The model under review builds one solid part; all positions refer to its coordinate system, in mm. A direction names the side the tool comes from. Coordinates: 2 decimals unless noted, no trailing zeros. Loops run counter-clockwise (first coordinate to the right, second up) from the corner with the lowest first, then second, coordinate; pieces in that order, holes last. Notation, with made-up numbers: M 8.25,80.5 L 58.25,80.5 A22 ccw 58.25,100.5 Z; hole C -18,89.25 d6. An arc over 180 degrees is marked long. Return JSON: item names as keys, results as strings.
```python
from build123d import *

# Parameters (mm, degrees)
SZKIC1_R                    = 7
DODANIE_WYCI_GNI_CIE1_DEPTH = 28
WYTNIJ_WYCI_GNI_CIE1_DEPTH  = 30.69848481


with BuildPart() as part:
    # Szkic1 → Dodanie-wyciągnięcie1 (new body)
    with BuildSketch(Plane.XY):
        Circle(SZKIC1_R)
        Polygon((4.922995461, 0.874137115), (1.704472782, 4.700507689), (-3.218522678, 3.826370574), (-4.922995461, -0.874137115), (-1.704472782, -4.700507689), (3.218522678, -3.826370574), align=None, mode=Mode.SUBTRACT)
    extrude(amount=DODANIE_WYCI_GNI_CIE1_DEPTH)

    # Szkic2 → Wytnij-wyciągnięcie1 (cut, through all)
    with BuildSketch(Plane.XY.offset(28)):
        Polygon((-3.423048557, 4.978226449), (1.499946904, 5.852363564), (1.23770577, 7.329262202), (-3.685289691, 6.455125087), align=None)
    extrude(amount=-WYTNIJ_WYCI_GNI_CIE1_DEPTH, mode=Mode.SUBTRACT)


solid = part.part
```
1. To check wall thickness, follow line 1 (Y direction, x = 0.5, z = 21.5); line 2 (X direction, y = -3.5, z = 13); line 3 (Y direction, x = 2.25, z = 9.5). State the ranges of each line that lie inside material, in increasing order.
Check values:
{"line 1": "-6.98 to -4.31, 4.49 to 5.67", "line 2": "-6.06 to -2.71, 3.34 to 6.06", "line 3": "-6.63 to -4, 4.05 to 6.63"}
2. Add section C-C on y = 1.25. Give the boundary of the cut face in (x, z).
Check values:
{"outline": "M -6.89,0 L -4.15,0 L -4.15,28 L -6.89,28 Z; M 4.61,0 L 6.89,0 L 6.89,28 L 4.61,28 Z"}
3. Add section B-B on x = 0. Give the boundary of the cut face in (y, z), plus the area to 3 significant figures.
Check values:
{"outline": "M -7,0 L -4.4,0 L -4.4,28 L -7,28 Z; M 4.4,0 L 5.59,0 L 5.59,28 L 4.4,28 Z", "area": "106 mm²"}
4. Add section A-A on z = 4. Give the boundary of the cut face in (x, y).
Check values:
{"outline": "M -3.6,6 A7 ccw long 1.32,6.87 L 1.5,5.85 L -3.42,4.98 Z; hole M -4.92,-0.87 L -1.7,-4.7 L 3.22,-3.83 L 4.92,0.87 L 1.7,4.7 L -3.22,3.83 Z"}
5. Insertion check: pin 1 Ø5 at (x, z) = (-1.5, 12) entering from +Y; pin 2 Ø1.5 at (x, z) = (0.5, 17) entering from -Y; pin 3 Ø4 at (x, z) = (3.5, 12) entering from +Y; pin 4 Ø1 at (x, z) = (3.5, 13.5) entering from -Y. Each pin has a flat end and moves straight along its axis. Give the tip position at first contact, or say it passes through.
Check values:
{"pin 1": "y = 6", "pin 2": "y = -7", "pin 3": "y = 6.84", "pin 4": "y = -6.32"}
6. The part is to be moulded in two halves that separate along Y. For faces 1 (the face through (0.955, -6.935, 13.804)), 2 (the face through (4.06, -1.51, 13.8)), 3 (the face through (0, -5, 0)), 4 (the face through (-3.515, 5.497, 14.196)), say which applies: released by +Y, released by -Y, zero draft, split by the parting line, or undercut.
Check values:
{"face 1": "split by the parting line", "face 2": "undercut", "face 3": "zero draft", "face 4": "released by +Y"}
7. Add section D-D on x = 5.5. Give the boundary of the cut face in (y, z), plus the area to 3 significant figures.
Check values:
{"outline": "M -4.33,0 L 4.33,0 L 4.33,28 L -4.33,28 Z", "area": "242 mm²"}
8. Machinability: for faces 5 (the face through (0, -5, 28)), 6 (the face through (-3.336, -2.761, 13.804)), which of the approach directions +Z, -Z, +X, -X, +Y, -Y give a long, thin tool a straight path to every point of the face, cutting with its end or side? Answer none if there is none.
Check values:
{"face 5": "+Z, +X, -X, +Y, -Y", "face 6": "+Z, -Z"}
